Autodesk Inventor part; units mm, degrees
ref_plane "YZ Plane" through (0, 0, 0) normal (1, 0, 0) x (0, 1, 0)
ref_plane "XZ Plane" through (0, 0, 0) normal (0, 1, 0) x (-1, 0, 0)
ref_plane "XY Plane" through (0, 0, 0) normal (0, 0, 1) x (1, 0, 0)
sketch "Sketch1" plane through (0, 0, 0) normal (1, 0, 0) x (0, 1, 0)
  arc A0 (0, -11) -> (0, 11) centre (0, 0) ccw
  arc A1 (0, -13) -> (0, 13) centre (0, 0) ccw
  line L0 (0, 13) -> (-16.0086, 13)
  line L1 (0, 11) -> (-18.0086, 11)
  line L2 (0, 0) -> (4.4908, 0)
  line L3 (-18.0086, 11) -> (-11, 11)
  line L4 (-16.0086, 13) -> (-16.0086, 33)
  line L5 (-16.0086, 33) -> (-18.0086, 33)
  line L6 (-18.0086, 33) -> (-18.0086, 11)
  line L7 (0, -13) -> (-16.0086, -13)
  line L8 (0, -11) -> (-18.0086, -11)
  line L9 (-18.0086, -11) -> (-11, -11)
  line L10 (-16.0086, -13) -> (-16.0086, -33)
  line L11 (-16.0086, -33) -> (-18.0086, -33)
  line L12 (-18.0086, -33) -> (-18.0086, -11)
  point P0 (-6.9282, 11)
  point P1 (-6.9282, -11)
  dimension "d0" = 22
  dimension "d1" = 2
  dimension "d12" = 18.0086
  dimension "d13" = 2
  dimension "d14" = 22
extrude "Extrusion1" add sketch "Sketch1" along normal blind 15
fillet "Fillet1" radius 2 2 edges at (7.5, -18.0086, -11) (7.5, -18.0086, 11)
fillet "Fillet2" radius 1 2 edges at (7.5, -16.0086, 13) (7.5, -16.0086, -13)
fillet "Fillet3" radius 3 4 edges at (15, -17.0086, 33) (0, -17.0086, 33) (15, -17.0086, -33) (0, -17.0086, -33)
sketch "Sketch2" plane through (0, -16.0086, 14) normal (0, 1, 0) x (1, 0, 0)
  circle A0 centre (7.5, -11) radius 3
  line L0 (3, -19) -> (12, -19)
  line L1 (0, 14) -> (27.6341, 14)
  circle A1 centre (7.5, 39) radius 3
  dimension "d8" = 6
  dimension "d9" = 8
extrude "Extrusion2" cut sketch "Sketch2" against normal blind 15
properties part number "rackbracket"
Input: part model. Units: mm. Frame: model coordinates. A direction names the side the tool comes from. Give positions to 0.01 mm unless a question says otherwise; leave off trailing zeros. Write each loop counter-clockwise with the first axis right and the second up, starting at its lowest first coordinate (ties: lowest second). Pieces come first, ordered by that corner, then holes. Notation, with made-up numbers: (-24.75, 4) - (32.25, 4) arc R21 cw to (32.25, 39) - close; hole circle Ø6 at (21, -14). An arc over 180 degrees is marked (long way). Write item = value, one per line. Start each with the question number.
1) Cut plane B-B (x = 7.5). Return loops of the section in (y, z).
2) Material intervals for L1, parallel to Z at x = 9, y = -4; L2, parallel to X at y = -17.25, z = -25; L3, parallel to Z at x = 7.5, y = -17.4, sorted ascending. Write a range as [from, to].
3) Reachability of faces 5 (the face through (7, -7, -13)), 6 (the face through (7.605, -17.438, 11.601)), 7 (the face through (7, -7, 13)) from +Z, -Z, +X, -X, +Y, -Y: full face, straight path, thin tool, end or side. Return the list, or none.
4) Draft query along X for faces 1 (the face through (10.27, -16.99, -23.85)), 2 (the face through (14.1, -17.02, -32.14)), 3 (the face through (10.27, -16.99, 26.15)), 4 (the face through (7, -16.009, -21)). Return one class per face: pulls with the +X half, pulls with the -X half, needs draft (parallel to the pull), parting line crosses it, or undercut.
5) Cut plane D-D (z = 0). Return loops of the section in (x, y).
6) Cut plane C-C (z = 25). Return loops of the section in (x, y), and give its area (3 significant figures).
7) Pin query (flat end, axial travel): pin 1 (12 mm diameter, centred on y = -14.5, z = 6.5, fed in from -X); pin 2 (8 mm diameter, centred on x = 9, y = 7, fed in from +Z); pin 3 (4.5 mm diameter, centred on x = 7.5, z = -27, fed in from +Y); pin 4 (6 mm diameter, centred on x = 10.5, y = -2.5, fed in from -Z). Return the tip coordinate at first contact, or that it passes through.
8) Cut plane A-A (y = -13). Return loops of the section in (x, z).
Answers follow:
q1.outline = (-18.01, -33) - (-16.01, -33) - (-16.01, -28) - (-18.01, -28) - close; (-18.01, -22) - (-16.01, -22) - (-16.01, -14) arc R1 cw to (-15.01, -13) - (0, -13) arc R13 ccw to (0, 13) - (-15.01, 13) arc R1 cw to (-16.01, 14) - (-16.01, 22) - (-18.01, 22) - (-18.01, 13) arc R2 ccw to (-16.01, 11) - (0, 11) arc R11 cw to (0, -11) - (-16.01, -11) arc R2 ccw to (-18.01, -13) - close; (-18.01, 28) - (-16.01, 28) - (-16.01, 33) - (-18.01, 33) - close
q2.L1 = [-13, -11], [11, 13]
q2.L2 = [0, 4.5], [10.5, 15]
q2.L3 = [-33, -28], [-22, -11.56], [11.56, 22], [28, 33]
q3.face_5 = -Z, +X, -X, +Y
q3.face_6 = +X, -X, -Y
q3.face_7 = +Z, +X, -X, +Y
q4.face_1 = undercut
q4.face_2 = pulls with the +X half
q4.face_3 = undercut
q4.face_4 = needs draft
q5.outline = (0, 11) - (15, 11) - (15, 13) - (0, 13) - close
q6.outline = (0, -18.01) - (4.5, -18.01) - (4.5, -16.01) - (0, -16.01) - close; (10.5, -18.01) - (15, -18.01) - (15, -16.01) - (10.5, -16.01) - close
q6.area = 18.0 mm^2
q7.pin_1 = 0
q7.pin_2 = 12.65
q7.pin_3 = -16.01
q7.pin_4 = -13
q8.outline = (0, -13) - (15, -13) - (15, -11) - (0, -11) - close; (0, 11) - (15, 11) - (15, 13) - (0, 13) - close
